Check sheet for the modelled part. Datum: model origin and axes. Units: mm. Face numbers are marked on the shaded views. Round coordinates to 2 decimals unless told otherwise and drop trailing zeros. Order: outer loops, then holes, each group sorted by start corner. A loop starts at its lowest first (then second) coordinate and runs counter-clockwise, first axis right, second up.
(1) Mould release check, pull along X, two halves, no side actions. Record for the marked faces 1, 2 and 3: released by +X, released by -X, zero draft, split by the parting line, or undercut.
(2) Sectioned sample at D-D, the plane y = 23. Enter the section's corners in (x, z), and give its area (3 significant figures).
(3) Sectioned sample at B-B, the plane x = 125. Enter the section's corners in (y, z).
(4) Thickness scan on probe 1 along Y at (x, z) = (22, 14.25); probe 2 along X at (y, z) = (8, 13); probe 3 along Z at (x, y) = (206, 8.5). Record the ranges inside material, lowest first.
(5) Sectioned sample at C-C, the plane x = 177. Enter the section's corners in (y, z).
(6) Depth check by flat-ended pin: pin 1 (4 mm diameter, centred on x = 104.91, z = 19.05, fed in from +Y). Enter the tip coordinate at first touch or a pass-through.
(7) Sectioned sample at A-A, the plane y = 46.5. Enter the section's corners in (x, z).
```python
from build123d import *

# Parameters (mm, degrees)
F0_W      = 304.8
F0_H      = 101.6
F1_DEPTH  = 25.4
F2_W      = 127
F2_H      = 25.4
F3_DEPTH  = 1.524
F4_W      = 254
F4_H      = 9.8806431205
F5_DEPTH  = 12.7
F7_DEPTH  = 12.7
F9_D      = 5.1054
F9_DEPTH  = 25.4
F9_TIP    = 1.5338169022
F11_D     = 5.1054
F11_DEPTH = 28.448
F11_TIP   = 1.5338169022


with BuildPart() as f1:
    # F0 (on Top) → F1 (new body)
    with BuildSketch(Plane.XY):
        with Locations((104.9140337646, 27.7402723759)):
            Rectangle(F0_W, F0_H)
    extrude(amount=F1_DEPTH)

    # F2 (on face) → F3 (cut)
    with BuildSketch(Plane.XY.offset(25.4)):
        with Locations((104.9140337646, 27.7402723759)):
            Rectangle(F2_W, F2_H)
    extrude(amount=-F3_DEPTH, mode=Mode.SUBTRACT)

    # F4 (on face) → F5 (cut)
    with BuildSketch(Plane.XY.offset(25.4)):
        with Locations((104.9140337646, 45.3805939362)):
            Rectangle(F4_W, F4_H)
    extrude(amount=-F5_DEPTH, mode=Mode.SUBTRACT)

    # F6 (on face) → F7 (cut)
    with BuildSketch(Plane.XY.offset(25.4)):
        Polygon((41.4140337646, 15.0402723759), (-22.0859662354, 15.0402723759), (-22.0859662354, 2.3402723759), (231.9140337646, 2.3402723759), (231.9140337646, 15.0402723759), (168.4140337646, 15.0402723759), align=None)
    extrude(amount=-F7_DEPTH, mode=Mode.SUBTRACT)

    # F9
    with Locations(Plane.XZ.offset(23.0597276241)):
        with Locations((104.9140337646, 19.05)):
            Hole(F9_D / 2, depth=F9_DEPTH)
            with Locations((0, 0, -(F9_DEPTH + F9_TIP / 2))):  # 118° drill point
                Cone(0, F9_D / 2, F9_TIP, mode=Mode.SUBTRACT)

    # F11
    with Locations(Plane(origin=(0, 78.5402723759, 0), x_dir=(-1, 0, 0), z_dir=(0, 1, 0))):
        with Locations((-104.9140337646, 19.05)):
            Hole(F11_D / 2, depth=F11_DEPTH)
            with Locations((0, 0, -(F11_DEPTH + F11_TIP / 2))):  # 118° drill point
                Cone(0, F11_D / 2, F11_TIP, mode=Mode.SUBTRACT)


solid = f1.part
```
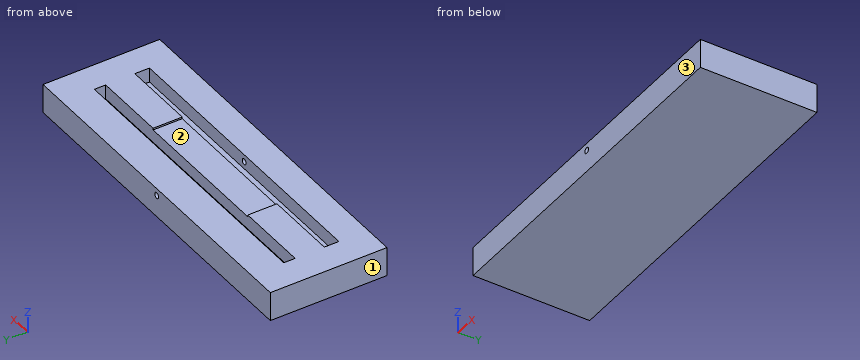
Derived:
1. face 1: released by -X
1. face 2: undercut
1. face 3: zero draft
2. outline: (-47.49, 0) - (257.31, 0) - (257.31, 25.4) - (168.41, 25.4) - (168.41, 23.88) - (41.41, 23.88) - (41.41, 25.4) - (-47.49, 25.4) - close
2. area: 7,550 mm2
3. outline: (-23.06, 0) - (78.54, 0) - (78.54, 25.4) - (50.32, 25.4) - (50.32, 12.7) - (40.44, 12.7) - (40.44, 23.88) - (15.04, 23.88) - (15.04, 12.7) - (2.34, 12.7) - (2.34, 25.4) - (-23.06, 25.4) - close
4. probe 1: y = -23.06 to 2.34, 15.04 to 40.44, 50.32 to 78.54
4. probe 2: x = -47.49 to -22.09, 231.91 to 257.31
4. probe 3: z = 0 to 12.7
5. outline: (-23.06, 0) - (78.54, 0) - (78.54, 25.4) - (50.32, 25.4) - (50.32, 12.7) - (40.44, 12.7) - (40.44, 25.4) - (15.04, 25.4) - (15.04, 12.7) - (2.34, 12.7) - (2.34, 25.4) - (-23.06, 25.4) - close
6. pin 1: stops at y = 40.44
7. outline: (-47.49, 0) - (257.31, 0) - (257.31, 25.4) - (231.91, 25.4) - (231.91, 12.7) - (-22.09, 12.7) - (-22.09, 25.4) - (-47.49, 25.4) - close
